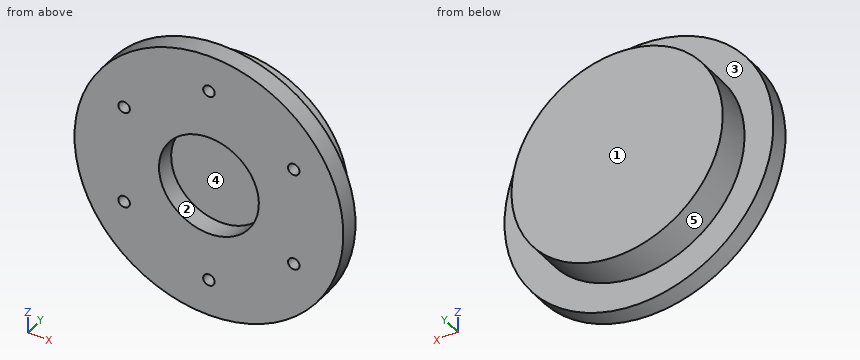
```python
from build123d import *

# Parameters (mm, degrees)
SKETCH1_R           = 35
SKETCH1_R_2         = 1.5
SKETCH1_R_3         = 13
BOSS_EXTRUDE1_DEPTH = 5
SKETCH2_R           = 27.5
BOSS_EXTRUDE2_DEPTH = 9


with BuildPart() as part:
    # Sketch1 → Boss-Extrude1 (new body)
    with BuildSketch(Plane(origin=(0, 0, 0), x_dir=(1, 0, 0), z_dir=(0, 1, 0))):
        with Locations(Location((0, 0, 0), (0, 0, 270))):
            Circle(SKETCH1_R)
        with Locations(Location((0, 25.5, 0), (0, 0, 270))):
            Circle(SKETCH1_R_2, mode=Mode.SUBTRACT)
        with Locations(Location((22.083647797, 12.75, 0), (0, 0, 270))):
            Circle(SKETCH1_R_2, mode=Mode.SUBTRACT)
        with Locations(Location((22.083647797, -12.75, 0), (0, 0, 270))):
            Circle(SKETCH1_R_2, mode=Mode.SUBTRACT)
        with Locations(Location((0, -25.5, 0), (0, 0, 270))):
            Circle(SKETCH1_R_2, mode=Mode.SUBTRACT)
        with Locations(Location((-22.083647797, -12.75, 0), (0, 0, 270))):
            Circle(SKETCH1_R_2, mode=Mode.SUBTRACT)
        with Locations(Location((-22.083647797, 12.75, 0), (0, 0, 270))):
            Circle(SKETCH1_R_2, mode=Mode.SUBTRACT)
        with Locations(Location((0, 0, 0), (0, 0, 270))):
            Circle(SKETCH1_R_3, mode=Mode.SUBTRACT)
    extrude(amount=BOSS_EXTRUDE1_DEPTH)

    # Sketch2 → Boss-Extrude2 (add)
    with BuildSketch(Plane(origin=(0, 5, 0), x_dir=(1, 0, 0), z_dir=(0, 1, 0))):
        with Locations(Location((0, 0, 0), (0, 0, 270))):
            Circle(SKETCH2_R)
    extrude(amount=BOSS_EXTRUDE2_DEPTH)


solid = part.part
```
The listing builds one solid part. Answer for the finished solid, in the listing's coordinates (mm). Face numbers are marked on the shaded views. A direction names the side the tool comes from. Give positions to 0.01 mm unless a question says otherwise; leave off trailing zeros. Order: outer loops, then holes, each group sorted by start corner. A loop starts at its lowest first (then second) coordinate and runs counter-clockwise, first axis right, second up. Notation, with made-up numbers: M 53.5,46.5 L 78.5,46.5 A30 ccw 78.5,71.5 Z; hole C 74.25,37.25 d8. An arc over 180 degrees is marked long. Put each result on its own line as item: value. Start each with the question number.
Item 1: The part is cut by section C-C, the plane y = 3.5. Determine the outline of the cut face in (x, z), and give its area (3 significant figures).
Item 2: Find the intervals of material crossed by line 1 along Y through (x, z) = (-20, 26); line 2 along X through (y, z) = (3.25, -26.5); line 3 along Y through (x, z) = (11, -2), in increasing order.
Item 3: Which of the six approach directions +Z, -Z, +X, -X, +Y, -Y give full straight-line access (tool end or side, diameter ignored) to the marked faces 1 and 2?
Item 4: The part is cut by section B-B, the plane x = -11. Determine the outline of the cut face in (y, z).
Item 5: The part is cut by section D-D, the plane y = 11.5. Determine the outline of the cut face in (x, z).
Item 6: Flat-ended cylindrical pins translate along their axes: P1, Ø2.5, axis at x = -22.08, z = -12.75, coming from the -Y side; P2, Ø2, axis at x = 2.5, y = 6.5, coming from the +Z side; P3, Ø1, axis at y = 1.5, z = -15, coming from the +X side. Find the tip coordinate at first contact, or state that the pin passes through.
Item 7: For a pull along X with two mould halves and no side action, classify the marked faces 3, 4 and 5 as +X half, -X half, draft (parallel to the pull), parting line (faces both ways), or undercut.
Item 8: The part is cut by section A-A, the plane z = 0. Determine the outline of the cut face in (x, y), and give its area (3 significant figures).
Answer key:
1. outline: C 0,0 d70; hole C -22.08,-12.75 d3; hole C -22.08,12.75 d3; hole C 0,0 d26; hole C 0,-25.5 d3; hole C 0,25.5 d3; hole C 22.08,-12.75 d3; hole C 22.08,12.75 d3
1. area: 3,280 mm²
2. line 1: y = 0 to 5
2. line 2: x = -22.86 to -1.12, 1.12 to 22.86
2. line 3: y = 5 to 14
3. face 1: +Z, -Z, +X, -X, +Y
3. face 2: -Y
4. outline: M 0,-33.23 L 5,-33.23 L 5,-25.2 L 14,-25.2 L 14,25.2 L 5,25.2 L 5,33.23 L 0,33.23 L 0,6.93 L 5,6.93 L 5,-6.93 L 0,-6.93 Z
5. outline: C 0,0 d55
6. P1: stops at y = 5
6. P2: stops at z = 27.46
6. P3: stops at x = 31.86
7. face 3: draft
7. face 4: undercut
7. face 5: parting line
8. outline: M -35,0 L -13,0 L -13,5 L 13,5 L 13,0 L 35,0 L 35,5 L 27.5,5 L 27.5,14 L -27.5,14 L -27.5,5 L -35,5 Z
8. area: 715 mm²
